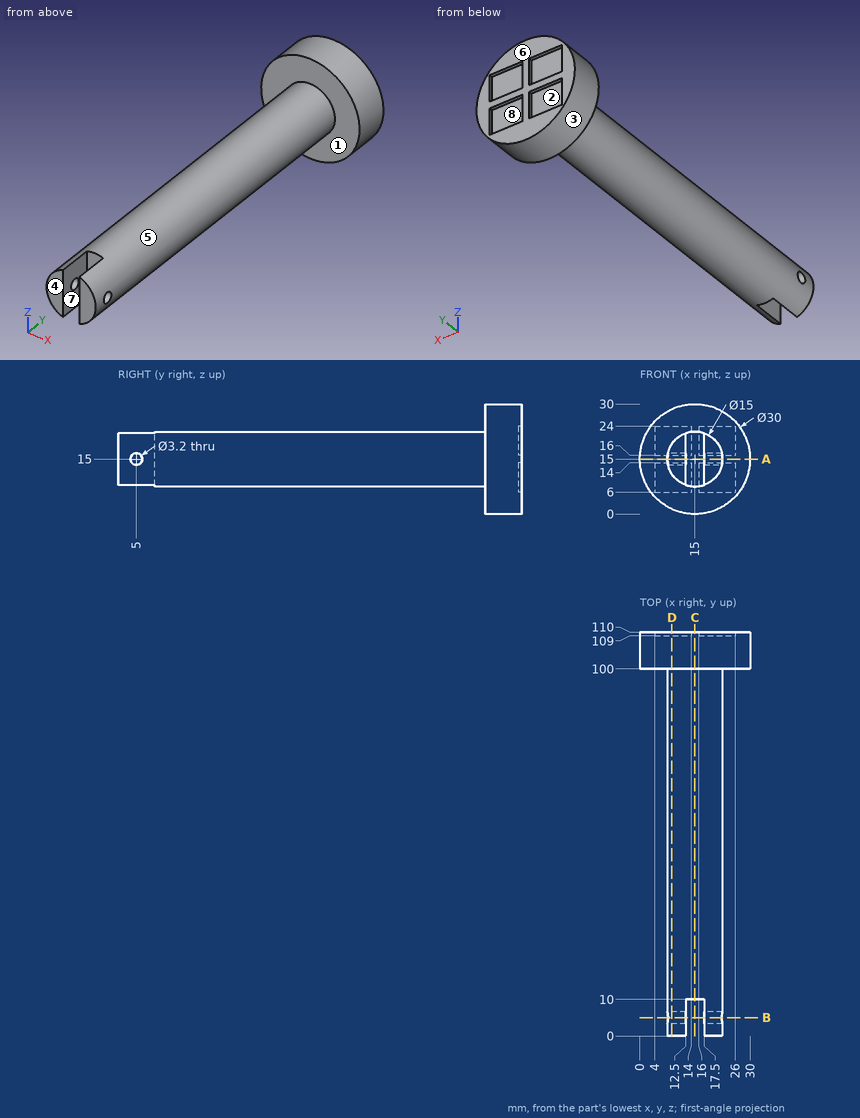
Verification items for this drawing (mm, ordinates from the low corner). A direction names the side the tool comes from. Coordinates: 2 decimals unless noted, no trailing zeros. Order: outer loops, then holes, each group sorted by start corner. A loop starts at its lowest first (then second) coordinate and runs counter-clockwise, first axis right, second up. Notation, with made-up numbers: (58, 39.5) -> (71, 39.5) arc R29 cw to (71, 61.5) -> close; hole circle Ø2 at (-34.75, 87). An arc over 180 degrees is marked (long way). Answer as CSV lines item,"result". Start each with the question number.
1) Material ranges on L1, parallel to Y at x = 19.35, z = 15; L2, parallel to Y at x = 16.75, z = 4; L3, parallel to Y at x = 14.75, z = 18.75, recorded low to high. Write a range as [from, to].
2) Set-up check for the marked faces 4, 5, 6, 7 and 8: record each of +Z, -Z, +X, -X, +Y, -Y from which the full face is reachable in a straight line by a thin tool's end or side.
3) Cross-section at A-A, the plane z = 15. Record the boundary of the cut face in (x, y), then the cut area to 3 significant figures.
4) Gauge pin test, flat ends, axial feed: pin 1 Ø4 at (x, y) = (8, 19) entering from -Z; pin 2 Ø2 at (x, z) = (7.5, 8.5) entering from -Y; pin 3 Ø2.5 at (x, z) = (11, 19.5) entering from +Y. Record the tip position at first contact, or that the pin passes through.
5) Cross-section at B-B, the plane y = 5. Record the boundary of the cut face in (x, z), then the cut area to 3 significant figures.
6) Cross-section at D-D, the plane x = 8.75. Record the boundary of the cut face in (y, z).
7) Release check for a two-part mould opening along Z. For the marked faces 1, 2 and 3 record: released by +Z, released by -Z, zero draft, split by the parting line, or undercut.
8) Cross-section at C-C, the plane x = 15. Record the boundary of the cut face in (y, z), then the cut area to 3 significant figures.
Conclusion:
1,L1,"y = [0, 3.4], [6.6, 110]"
1,L2,"y = [100, 110]"
1,L3,"y = [10, 110]"
2,face 4,"+Z, -Z, +X, -X, -Y"
2,face 5,"-Y"
2,face 6,"+Z, -Z, +X, -X, +Y"
2,face 7,"+Z, -Z, -Y"
2,face 8,"+Y"
3,outline,"(0, 100) -> (7.5, 100) -> (7.5, 6.6) -> (12.5, 6.6) -> (12.5, 10) -> (17.5, 10) -> (17.5, 6.6) -> (22.5, 6.6) -> (22.5, 100) -> (30, 100) -> (30, 110) -> (0, 110) -> close; (7.5, 0) -> (12.5, 0) -> (12.5, 3.4) -> (7.5, 3.4) -> close; (17.5, 0) -> (22.5, 0) -> (22.5, 3.4) -> (17.5, 3.4) -> close"
3,area,"1,720 mm²"
4,pin 1,"stops at z = 9.41"
4,pin 2,"stops at y = 100"
4,pin 3,"stops at y = 109"
5,outline,"(7.67, 13.4) arc R7.5 ccw to (12.5, 7.93) -> (12.5, 13.4) -> close; (7.67, 16.6) -> (12.5, 16.6) -> (12.5, 22.07) arc R7.5 ccw to start; (17.5, 7.93) arc R7.5 ccw to (22.33, 13.4) -> (17.5, 13.4) -> close; (17.5, 16.6) -> (22.33, 16.6) arc R7.5 ccw to (17.5, 22.07) -> close"
5,area,"71.5 mm²"
6,outline,"(0, 10.85) -> (100, 10.85) -> (100, 1.36) -> (110, 1.36) -> (110, 6) -> (109, 6) -> (109, 14) -> (110, 14) -> (110, 16) -> (109, 16) -> (109, 24) -> (110, 24) -> (110, 28.64) -> (100, 28.64) -> (100, 19.15) -> (0, 19.15) -> close; hole circle Ø3.2 at (5, 15)"
7,face 1,"zero draft"
7,face 2,"undercut"
7,face 3,"split by the parting line"
8,outline,"(10, 7.5) -> (100, 7.5) -> (100, 0) -> (110, 0) -> (110, 30) -> (100, 30) -> (100, 22.5) -> (10, 22.5) -> close"
8,area,"1,650 mm²"
